Check sheet for the modelled part. Datum: model origin and axes. Units: mm. A direction names the side the tool comes from. Round coordinates to 2 decimals unless told otherwise and drop trailing zeros. Write each loop counter-clockwise with the first axis right and the second up, starting at its lowest first coordinate (ties: lowest second). Pieces come first, ordered by that corner, then holes. Notation, with made-up numbers: (-12, -1.5) -> (23, -1.5) arc R24 ccw to (23, 26.5) -> close; hole circle Ø3 at (65, 87). An arc over 180 degrees is marked (long way). One line per item, written item: value.
from build123d import *

# Parameters (mm, degrees)
F1_DEPTH      = 635
F3_DEPTH      = 22
F4_W          = 100
F4_H          = 100
F5_DEPTH      = 10
F6_R          = 11
F7_DEPTH      = 8
F7_DEPTH_BACK = 63.001
F9_DEPTH      = 50.001
F9_DEPTH_BACK = 50.001
F10_R         = 10
F11_DEPTH     = 200


with BuildPart() as f1:
    # F0 (on Right) → F1 (new body, symmetric)
    with BuildSketch(Plane.YZ):
        with BuildLine():
            Line((90, 42), (90, 50))
            Line((90, 50), (28, 50))
            ThreePointArc((28, 50), (8.2010101268, 41.7989898732), (0, 22))
            Line((0, 22), (0, -22))
            ThreePointArc((0, -22), (8.2010101268, -41.7989898732), (28, -50))
            Line((28, -50), (90, -50))
            Line((90, -50), (90, -42))
            Line((90, -42), (28, -42))
            ThreePointArc((28, -42), (13.8578643763, -36.1421356237), (8, -22))
            Line((8, -22), (8, 22))
            ThreePointArc((8, 22), (13.8578643763, 36.1421356237), (28, 42))
            Line((28, 42), (90, 42))
        make_face()
    extrude(amount=F1_DEPTH, both=True)

    # F2 (on Top) → F3 (join, symmetric)
    with BuildSketch(Plane.XY):
        Polygon((-80, 0), (-143, 0), (-143, -5), (-85, -5), (-85, -63), (-80, -63), align=None)
        Polygon((80, -63), (85, -63), (85, -5), (143, -5), (143, 0), (80, 0), align=None)
    extrude(amount=F3_DEPTH, both=True)

    # F4 (on face) → F5 (join)
    with BuildSketch(Plane(origin=(0, 90, 0), x_dir=(-1, 0, 0), z_dir=(0, 1, 0))):
        with Locations((-135, 0)):
            Rectangle(F4_W, F4_H)
        with Locations((135, 0)):
            Rectangle(F4_W, F4_H)
    extrude(amount=F5_DEPTH)

    # F6 (on Front) → F7 (cut, two sides)
    with BuildSketch(Plane.XZ) as f7_sk:
        with Locations((-115, 0)):
            Circle(F6_R)
        with Locations((115, 0)):
            Circle(F6_R)
    extrude(amount=-F7_DEPTH, mode=Mode.SUBTRACT)
    extrude(f7_sk.sketch, amount=F7_DEPTH_BACK, mode=Mode.SUBTRACT)

    # F8 (on Top) → F9 (cut, two sides)
    with BuildSketch(Plane.XY) as f9_sk:
        with BuildLine():
            Line((-590, 57.5), (-590, 62.5))
            ThreePointArc((-590, 62.5), (-600, 72.5), (-610, 62.5))
            Line((-610, 62.5), (-610, 57.5))
            ThreePointArc((-610, 57.5), (-600, 47.5), (-590, 57.5))
        make_face()
        with BuildLine():
            ThreePointArc((610, 62.5), (600, 72.5), (590, 62.5))
            Line((590, 62.5), (590, 57.5))
            ThreePointArc((590, 57.5), (600, 47.5), (610, 57.5))
            Line((610, 57.5), (610, 62.5))
        make_face()
    extrude(amount=F9_DEPTH, mode=Mode.SUBTRACT)
    extrude(f9_sk.sketch, amount=-F9_DEPTH_BACK, mode=Mode.SUBTRACT)

    # F10 (on face) → F11 (join)
    with BuildSketch(Plane.XZ.offset(-90)):
        with Locations((-115, 0)):
            Circle(F10_R)
        with Locations((115, 0)):
            Circle(F10_R)
    extrude(amount=F11_DEPTH)


solid = f1.part
Item 1: Sectioned sample at C-C on y = -89. Enter the section's corners in (x, z), and give its area (3 significant figures).
Answer:
outline: circle Ø20 at (-115, 0); circle Ø20 at (115, 0)
area: 628 mm^2
Item 2: Mould release check, pull along X, two halves, no side actions. Record for faces 6 (the cylindrical face through (-125, -9, 0)), 7 (the flat face through (392, 0, 0)), 8 (the cylindrical face through (104, 1, 0)): pulls with the +X half, pulls with the -X half, needs draft (parallel to the pull), parting line crosses it, or undercut.
Answer:
face 6: undercut
face 7: needs draft
face 8: undercut
Item 3: Sectioned sample at A-A on x = -157.5. Enter the section's corners in (y, z).
Answer:
outline: (0, -22) arc R28 ccw to (28, -50) -> (100, -50) -> (100, 50) -> (28, 50) arc R28 ccw to (0, 22) -> close; hole (8, -22) arc R20 ccw to (28, -42) -> (90, -42) -> (90, 42) -> (28, 42) arc R20 ccw to (8, 22) -> close
Item 4: Thickness scan on line 1 (Z direction, x = 115, y = -0.5); line 2 (Z direction, x = -252, y = 63.5); line 3 (Y direction, x = 150, z = 16.5). Record the ranges inside material, lowest first.
Answer:
line 1: z = -22 to -11, -10 to 10, 11 to 22
line 2: z = -50 to -42, 42 to 50
line 3: y = 0 to 8, 90 to 100
Item 5: Tool access check on faces 1 (the flat face through (83, -17, -22)), 2 (the flat face through (-98, -3, 22)), 3 (the flat face through (9, 59, 42)), 4 (the cylindrical face through (105, -9, 0)), 5 (the flat face through (-85, -34, 0)). Record the directions out of +Z, -Z, +X, -X, +Y, -Y that give a thin tool (end or side, any length) a straight path to the whole face; none if there is none.
Answer:
face 1: -Z, +X, -X, -Y
face 2: +Z, +X, -X, -Y
face 3: +X, -X
face 4: -Y
face 5: +Z, -Z, -Y
Item 6: Depth check by flat-ended pin: P1, Ø1, axis at x = 313.5, y = 18.5, coming from the +Z side; P2, Ø22, axis at x = 10, z = -9, coming from the -Y side; P3, Ø11, axis at y = 94.5, z = 23.5, coming from the -X side. Enter the tip coordinate at first touch or a pass-through.
Answer:
P1: stops at z = 48.51
P2: stops at y = 0
P3: stops at x = -185
Item 7: Sectioned sample at B-B on x = -515. Enter the section's corners in (y, z), and give its area (3 significant figures).
Answer:
outline: (0, -22) arc R28 ccw to (28, -50) -> (90, -50) -> (90, -42) -> (28, -42) arc R20 cw to (8, -22) -> (8, 22) arc R20 cw to (28, 42) -> (90, 42) -> (90, 50) -> (28, 50) arc R28 ccw to (0, 22) -> close
area: 1,950 mm^2
